Autodesk Inventor part; units mm, degrees
ref_plane "YZ Plane" through (0, 0, 0) normal (1, 0, 0) x (0, 1, 0)
ref_plane "XZ Plane" through (0, 0, 0) normal (0, 1, 0) x (-1, 0, 0)
ref_plane "XY Plane" through (0, 0, 0) normal (0, 0, 1) x (1, 0, 0)
sketch "Sketch1" plane through (0, 0, 0) normal (0, 1, 0) x (-1, 0, 0)
  circle A0 centre (0, 0) radius 6.35
  circle A1 centre (0, 0) radius 3.175
  dimension "d0" = 12.7
  dimension "d1" = 6.35
extrude "Extrusion1" add sketch "Sketch1" along normal blind 15.24 contours A1
extrude "Extrusion2" add sketch "Sketch1" against normal blind 1.27 contours A0 | A1
fillet "Fillet1" radius 1.5875 1 edges at (3.175, 0, 0)
properties part number "Pin_3DPrint"
Work out the finished part from the listing and answer in its coordinate system (mm). A direction names the side the tool comes from. Give positions to 0.01 mm unless a question says otherwise; leave off trailing zeros. Loops run counter-clockwise (first coordinate to the right, second up) from the corner with the lowest first, then second, coordinate; pieces in that order, holes last. Notation, with made-up numbers: (75, 73.5) -> (122, 73.5) arc R7 ccw to (122, 83.5) -> close; hole circle Ø4 at (11.5, 23). An arc over 180 degrees is marked (long way). Put each result on its own line as item: value. Start each with the question number.
Item 1: Which of the six approach directions +Z, -Z, +X, -X, +Y, -Y give full straight-line access (tool end or side, diameter ignored) to faces 1 (the face through (0, -1.27, 0)), 2 (the face through (0.69, 8.32, 3.1))?
Item 2: The part is cut by section D-D (z = -5.25). Give the vertices of the cut face in (x, y), then the cut area to 3 significant figures.
Item 3: Each of these flat-tipped pins is pushed along its axis until it touches: P1, Ø2, axis at x = -1.5, y = 3.5, coming from the -Z side; P2, Ø6, axis at x = -0.5, y = 12, coming from the -Z side (3 decimals); P3, Ø2, axis at y = 6.5, z = -1.5, coming from the +X side. Where does it stop, or does it pass through?
Item 4: Find the intervals of material crossed by L1, parallel to Y at x = 2, z = 4.25; L2, parallel to Z at x = -0.5, y = 2.25, in increasing order. Write a range as [from, to].
Item 5: The part is cut by section C-C (y = 11). Give the vertices of the cut face in (x, z) (3 decimals), then the cut area to 3 significant figures.
Answers below:
1. face 1: +Z, -Z, +X, -X, -Y
1. face 2: +Y
2. outline: (-3.57, -1.27) -> (3.57, -1.27) -> (3.57, 0) -> (-3.57, 0) -> close
2. area: 9.07 mm2
3. P1: z = -3.14
3. P2: z = -3.175
3. P3: x = 3.14
4. L1: [-1.27, 0]
4. L2: [-3.14, 3.14]
5. outline: circle Ø6.35 at (0, 0)
5. area: 31.7 mm2
